The listing builds one solid part. Answer for the finished solid, in the listing's coordinates (mm). Give positions to 0.01 mm unless a question says otherwise; leave off trailing zeros. Loops run counter-clockwise (first coordinate to the right, second up) from the corner with the lowest first, then second, coordinate; pieces in that order, holes last. Notation, with made-up numbers: M -29,86 L -1,86 A14 cw -1,105 Z; hole C 83.25,12 d1. An arc over 180 degrees is marked long. Use one line per item in the form item = value. Start each with the question number.
1. Each of these flat-tipped pins is pushed along its axis until it touches: pin 1 Ø1.5 at (x, z) = (11.5, 6.5) entering from -Y; pin 2 Ø8 at (y, z) = (-18.5, 11.5) entering from -X; pin 3 Ø15 at (x, y) = (0, 0) entering from -Z; pin 4 Ø10 at (x, z) = (-18.5, 17.5) entering from -Y. Where does it stop, or does it pass through?
2. The part is cut by section A-A (y = 0). Write down the section's boundary in (x, z), and give its area (3 significant figures).
3. Straight lines are drawn through the part: line 1 (Y direction, x = 0, z = 9.25); line 2 (X direction, y = 2, z = 19.5); line 3 (X direction, y = 1, z = 8). For each, find the intervals that lie inside material, in ascending order. Write a range as from..to.
4. The part is cut by section D-D (y = 21). Write down the section's boundary in (x, z), and give its area (3 significant figures).
5. The mould has two halves that part along X. Classify faces 1 (the face through (11.923, 3.755, 12.36)), 2 (the face through (-16.88, 16.68, 23.77)), 3 (the face through (15.3, 0.3, 25)): released by +X, released by -X, zero draft, split by the parting line, or undercut.
6. The part is cut by section C-C (z = 21.25). Write down the section's boundary in (x, y), and give its area (3 significant figures).
from build123d import *

# Parameters (mm, degrees)
SKETCH2_R      = 12.5
EXTRUDE2_DEPTH = 25
CHAMFER3_SIZE  = 2.5
CHAMFER4_SIZE  = 2.5


with BuildPart() as part:
    # Sketch2 → Extrude2 (new body)
    with BuildSketch(Plane.XY):
        Polygon((-25, 10.355339059), (-10.355339059, 25), (10.355339059, 25), (25, 10.355339059), (25, -10.355339059), (10.355339059, -25), (-10.355339059, -25), (-25, -10.355339059), align=None)
        Circle(SKETCH2_R, mode=Mode.SUBTRACT)
    extrude(amount=EXTRUDE2_DEPTH)

    # Chamfer3
    chamfer3_edges = [part.edges().sort_by_distance(p)[0] for p in [
        (-12.5, 0, 0),
        (17.67766953, 17.67766953, 0),
        (25, 0, 0),
        (17.67766953, -17.67766953, 0),
        (0, -25, 0),
        (-17.67766953, -17.67766953, 0),
        (-25, 0, 0),
        (-17.67766953, 17.67766953, 0),
        (0, 25, 0),
    ]]
    chamfer(chamfer3_edges, length=CHAMFER3_SIZE)

    # Chamfer4
    chamfer4_edges = [part.edges().sort_by_distance(p)[0] for p in [
        (-25, 0, 25),
        (-17.67766953, -17.67766953, 25),
        (0, -25, 25),
        (17.67766953, -17.67766953, 25),
        (-12.5, 0, 25),
        (25, 0, 25),
        (17.67766953, 17.67766953, 25),
        (0, 25, 25),
        (-17.67766953, 17.67766953, 25),
    ]]
    chamfer(chamfer4_edges, length=CHAMFER4_SIZE)


solid = part.part
Derived:
q1.pin_1 = -24.61
q1.pin_2 = -20.86
q1.pin_3 = through
q1.pin_4 = -21.86
q2.outline = M -25,2.5 L -22.5,0 L -15,0 L -12.5,2.5 L -12.5,22.5 L -15,25 L -22.5,25 L -25,22.5 Z; M 12.5,2.5 L 15,0 L 22.5,0 L 25,2.5 L 25,22.5 L 22.5,25 L 15,25 L 12.5,22.5 Z
q2.area = 600 mm2
q3.line_1 = -25..-12.5, 12.5..25
q3.line_2 = -25..-12.34, 12.34..25
q3.line_3 = -25..-12.46, 12.46..25
q4.outline = M -14.36,2.5 L -10.82,0 L 10.82,0 L 14.36,2.5 L 14.36,22.5 L 10.82,25 L -10.82,25 L -14.36,22.5 Z
q4.area = 700 mm2
q5.face_1 = undercut
q5.face_2 = released by -X
q5.face_3 = zero draft
q6.outline = M -25,-10.36 L -10.36,-25 L 10.36,-25 L 25,-10.36 L 25,10.36 L 10.36,25 L -10.36,25 L -25,10.36 Z; hole C 0,0 d25
q6.area = 1,580 mm2
